Could you check a few things on this model? Use its own coordinates, in mm. Face numbers are marked on the shaded views. A direction names the side the tool comes from. Give positions to 0.01 mm unless a question says otherwise; leave off trailing zeros. Order: outer loops, then holes, each group sorted by start corner. A loop starts at its lowest first (then second) coordinate and runs counter-clockwise, first axis right, second up. Notation, with made-up numbers: (51, 21) - (104, 21) arc R28 ccw to (104, 46) - close; hole circle Ø3 at (36.25, 69). An arc over 180 degrees is marked (long way). Put each result on its own line as item: value.
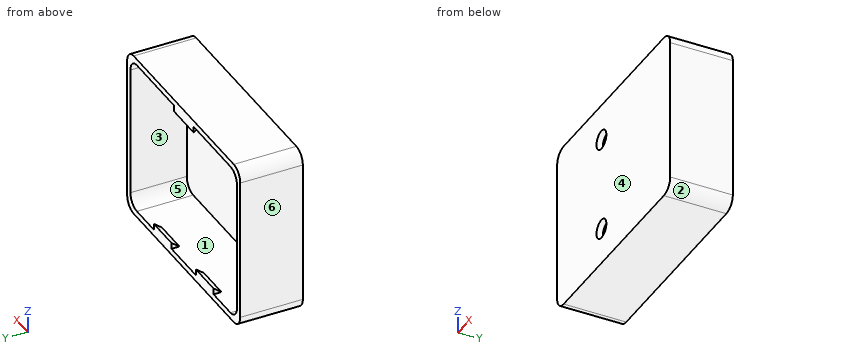
from build123d import *

# Parameters (mm, degrees)
SKETCH1_W           = 35
SKETCH1_H           = 27
BOSS_EXTRUDE1_DEPTH = 10
SKETCH2_W           = 33
SKETCH2_H           = 25
CUT_EXTRUDE1_DEPTH  = 9
SKETCH3_W           = 5.453863721
SKETCH3_H           = 1.273193124
BOSS_EXTRUDE2_DEPTH = 1
SKETCH4_W           = 6.116939674
SKETCH4_H           = 1.326628088
BOSS_EXTRUDE5_DEPTH = 1
CUT_EXTRUDE2_DEPTH  = 8
CUT_EXTRUDE5_DEPTH  = 8
CUT_EXTRUDE6_DEPTH  = 8
FILLET1_R           = 2
FILLET2_R           = 2
SKETCH8_R           = 1.524
CUT_EXTRUDE7_DEPTH  = 8


with BuildPart() as part:
    # Sketch1 → Boss-Extrude1 (new body)
    with BuildSketch(Plane(origin=(0, 0, 0), x_dir=(1, 0, 0), z_dir=(0, 1, 0))):
        Rectangle(SKETCH1_W, SKETCH1_H)
    extrude(amount=BOSS_EXTRUDE1_DEPTH)

    # Sketch2 → Cut-Extrude1 (cut)
    with BuildSketch(Plane(origin=(0, 10, 0), x_dir=(1, 0, 0), z_dir=(0, 1, 0))):
        Rectangle(SKETCH2_W, SKETCH2_H)
    extrude(amount=-CUT_EXTRUDE1_DEPTH, mode=Mode.SUBTRACT)

    # Sketch3 → Boss-Extrude2 (add)
    with BuildSketch(Plane.XY.offset(-12.5)):
        with Locations((6.508277375, 9.363403438)):
            Rectangle(SKETCH3_W, SKETCH3_H)
        with Locations((-6.508277375, 9.363403438)):
            Rectangle(SKETCH3_W, SKETCH3_H)
    extrude(amount=BOSS_EXTRUDE2_DEPTH)

    # Sketch4 → Boss-Extrude5 (add)
    with BuildSketch(Plane(origin=(0, 0, 12.5), x_dir=(-1, 0, 0), z_dir=(0, 0, -1))):
        with Locations((0, 9.336685956)):
            Rectangle(SKETCH4_W, SKETCH4_H)
    extrude(amount=BOSS_EXTRUDE5_DEPTH)

    # Sketch5 → Cut-Extrude2 (cut)
    with BuildSketch(Plane(origin=(3.058469837, 0, 0), x_dir=(0, 0, -1), z_dir=(1, 0, 0))):
        Polygon((-12.5, 8.673371912), (-11.5, 10), (-11.5, 8.673371912), align=None)
    extrude(amount=-CUT_EXTRUDE2_DEPTH, mode=Mode.SUBTRACT)

    # Sketch6 → Cut-Extrude5 (cut)
    with BuildSketch(Plane(origin=(9.235209235, 0, 0), x_dir=(0, 0, -1), z_dir=(1, 0, 0))):
        Polygon((11.5, 10), (12.5, 8.726806876), (11.5, 8.726806876), align=None)
    extrude(amount=-CUT_EXTRUDE5_DEPTH, mode=Mode.SUBTRACT)

    # Sketch7 → Cut-Extrude6 (cut)
    with BuildSketch(Plane(origin=(-3.781345514, 0, 0), x_dir=(0, 0, -1), z_dir=(1, 0, 0))):
        Polygon((11.5, 10), (12.5, 8.726806876), (11.5, 8.726806876), align=None)
    extrude(amount=-CUT_EXTRUDE6_DEPTH, mode=Mode.SUBTRACT)

    # Fillet1
    fillet1_edges = [part.edges().sort_by_distance(p)[0] for p in [
        (-17.5, 5, -13.5),
        (17.5, 5, -13.5),
        (17.5, 5, 13.5),
        (-17.5, 5, 13.5),
    ]]
    fillet(fillet1_edges, radius=FILLET1_R)

    # Fillet2
    fillet2_edges = [part.edges().sort_by_distance(p)[0] for p in [
        (-16.5, 5.5, 12.5),
        (-16.5, 5.5, -12.5),
        (16.5, 5.5, -12.5),
        (16.5, 5.5, 12.5),
    ]]
    fillet(fillet2_edges, radius=FILLET2_R)

    # Sketch8 → Cut-Extrude7 (cut)
    with BuildSketch(Plane(origin=(0, 1, 0), x_dir=(1, 0, 0), z_dir=(0, 1, 0))):
        with Locations(Location((-3.8, -7.62, 0), (0, 0, 270))):
            Circle(SKETCH8_R)
        with Locations(Location((-3.8, 7.62, 0), (0, 0, 270))):
            Circle(SKETCH8_R)
    extrude(amount=-CUT_EXTRUDE7_DEPTH, mode=Mode.SUBTRACT)


solid = part.part
1) Suppose I cut it at A-A, the plane z = -7.62. List the corners of the cut face in (x, y) for me.
Filled in:
outline: (-17.5, 0) - (-5.32, 0) - (-5.32, 1) - (-16.5, 1) - (-16.5, 10) - (-17.5, 10) - close; (-2.28, 0) - (17.5, 0) - (17.5, 10) - (16.5, 10) - (16.5, 1) - (-2.28, 1) - close
2) If I drill on line 1 (X direction, y = 8, z = 3.5); line 2 (X direction, y = 0.35, z = -7.62); line 3 (Z direction, x = -10.5, y = 6.5), over which ranges is the centre line in solid material (lowest first)? Write a range as [from, to].
Filled in:
line 1: x = [-17.5, -16.5], [16.5, 17.5]
line 2: x = [-17.5, -5.32], [-2.28, 17.5]
line 3: z = [-13.5, -12.5], [12.5, 13.5]
3) Suppose I cut it at C-C, the plane z = 1. List the corners of the cut face in (x, y) for me.
Filled in:
outline: (-17.5, 0) - (17.5, 0) - (17.5, 10) - (16.5, 10) - (16.5, 1) - (-16.5, 1) - (-16.5, 10) - (-17.5, 10) - close
4) Suppose I cut it at B-B, the plane y = 6.5. List the corners of the cut face in (x, z) for me.
Filled in:
outline: (-17.5, -11.5) arc R2 ccw to (-15.5, -13.5) - (15.5, -13.5) arc R2 ccw to (17.5, -11.5) - (17.5, 11.5) arc R2 ccw to (15.5, 13.5) - (-15.5, 13.5) arc R2 ccw to (-17.5, 11.5) - close; hole (-16.5, -10.5) arc R2 ccw to (-14.5, -12.5) - (14.5, -12.5) arc R2 ccw to (16.5, -10.5) - (16.5, 10.5) arc R2 ccw to (14.5, 12.5) - (-14.5, 12.5) arc R2 ccw to (-16.5, 10.5) - close
5) We'd pull the mould along Z, two halves only. Please class the marked faces 1, 2, 3 and 4: pulls with the +Z half, pulls with the -Z half, needs draft (parallel to the pull), parting line crosses it, or undercut.
Filled in:
face 1: undercut
face 2: pulls with the -Z half
face 3: undercut
face 4: needs draft
6) I'm going to push flat-ended pins straight in: pin 1 (0.5 mm diameter, centred on y = 9.5, z = 12, fed in from -X); pin 2 (1 mm diameter, centred on x = -11, z = -9, fed in from -Y); pin 3 (1.8 mm diameter, centred on x = -3.8, z = 7.62, fed in from -Y); pin 4 (0.8 mm diameter, centred on y = 9, z = 12, fed in from +X). Where does each tip first touch, or does it pass through?
Filled in:
pin 1: stops at x = -17.48
pin 2: stops at y = 0
pin 3: passes through
pin 4: stops at x = 17.5
7) Which directions (+Z, -Z, +X, -X, +Y, -Y) give clear straight access to the entire face, cutting with the end or side of a thin tool? Please do the marked faces 5 and 6.
Filled in:
face 5: +Y
face 6: +Z, -Z, -X, +Y, -Y
